Here's how the part is built. I have some questions about the finished solid (model axes, mm). Round coordinates to 2 decimals unless told otherwise and drop trailing zeros. Put each result on its own line as item: value. Start each with the question number.
1) Will this pin go through, and if not, where does the flat tip stop? P1, Ø2.5, axis at x = -86.21, z = 15.12, coming from the +Y side.
2) If I drill on line 1 along X through (y, z) = (-2.4, -26.5); line 2 along Z through (x, y) = (155, -0.95); line 3 along X through (y, z) = (-0.35, 70), over which ranges is the centre line in solid material (lowest first)? Write a range as [from, to].
3) I want a section at A-A, the plane y = -1.65. Give the number of separate pieces and of enclosed holes in the cut face, then the cut area to 3 significant figures.
from build123d import *

# Parameters (mm, degrees)
F0_R     = 1.89865
F1_DEPTH = 3.175


with BuildPart() as f1:
    # F0 (on Front) → F1 (new body)
    with BuildSketch(Plane.XZ):
        with BuildLine():
            Line((200.025, 95.25), (-200.025, 95.25))
            ThreePointArc((-200.025, 95.25), (-202.2700640303, 94.3200640303), (-203.2, 92.075))
            Line((-203.2, 92.075), (-203.2, -92.075))
            ThreePointArc((-203.2, -92.075), (-202.2700640303, -94.3200640303), (-200.025, -95.25))
            Line((-200.025, -95.25), (200.025, -95.25))
            ThreePointArc((200.025, -95.25), (202.2700640303, -94.3200640303), (203.2, -92.075))
            Line((203.2, -92.075), (203.2, 92.075))
            ThreePointArc((203.2, 92.075), (202.2700640303, 94.3200640303), (200.025, 95.25))
        make_face()
        with Locations((-152.4, -82.55)):
            Circle(F0_R, mode=Mode.SUBTRACT)
        with Locations((-101.6, -82.55)):
            Circle(F0_R, mode=Mode.SUBTRACT)
        with Locations((-150.2112307024, -64.8801388249)):
            Circle(F0_R, mode=Mode.SUBTRACT)
        with Locations((-50.8, -82.55)):
            Circle(F0_R, mode=Mode.SUBTRACT)
        with Locations((0, -82.55)):
            Circle(F0_R, mode=Mode.SUBTRACT)
        with BuildLine():
            ThreePointArc((-84.3125807024, -64.8801388249), (-86.2112307024, -66.7787888249), (-88.1098807024, -64.8801388249))
            ThreePointArc((-88.1098807024, -64.8801388249), (-86.2112307024, -62.9814888249), (-84.3125807024, -64.8801388249))
        make_face(mode=Mode.SUBTRACT)
        with BuildLine():
            ThreePointArc((-188.1665156039, -0.0463944584), (-187.2365796342, 2.1986695719), (-184.9915156039, 3.1286055416))
            Line((-184.9915156039, 3.1286055416), (-165.9415156039, 3.1286055416))
            ThreePointArc((-165.9415156039, 3.1286055416), (-163.6964515737, 2.1986695719), (-162.7665156039, -0.0463944584))
            Line((-162.7665156039, -0.0463944584), (-162.7665156039, -50.8463944584))
            ThreePointArc((-162.7665156039, -50.8463944584), (-163.6964515737, -53.0914584887), (-165.9415156039, -54.0213944584))
            Line((-165.9415156039, -54.0213944584), (-184.9915156039, -54.0213944584))
            ThreePointArc((-184.9915156039, -54.0213944584), (-187.2365796342, -53.0914584887), (-188.1665156039, -50.8463944584))
            Line((-188.1665156039, -50.8463944584), (-188.1665156039, -0.0463944584))
        make_face(mode=Mode.SUBTRACT)
        with BuildLine():
            ThreePointArc((-72.1112307024, 0.5198611751), (-71.1812947327, 2.7649252054), (-68.9362307024, 3.6948611751))
            Line((-68.9362307024, 3.6948611751), (-49.8862307024, 3.6948611751))
            ThreePointArc((-49.8862307024, 3.6948611751), (-47.6411666721, 2.7649252054), (-46.7112307024, 0.5198611751))
            Line((-46.7112307024, 0.5198611751), (-46.7112307024, -50.2801388249))
            ThreePointArc((-46.7112307024, -50.2801388249), (-47.6411666721, -52.5252028551), (-49.8862307024, -53.4551388249))
            Line((-49.8862307024, -53.4551388249), (-68.9362307024, -53.4551388249))
            ThreePointArc((-68.9362307024, -53.4551388249), (-71.1812947327, -52.5252028551), (-72.1112307024, -50.2801388249))
            Line((-72.1112307024, -50.2801388249), (-72.1112307024, 0.5198611751))
        make_face(mode=Mode.SUBTRACT)
        with Locations((50.8, -82.55)):
            Circle(F0_R, mode=Mode.SUBTRACT)
        with Locations((101.6, -82.55)):
            Circle(F0_R, mode=Mode.SUBTRACT)
        with Locations((62.75, -63.5)):
            Circle(F0_R, mode=Mode.SUBTRACT)
        with Locations((152.4, -82.55)):
            Circle(F0_R, mode=Mode.SUBTRACT)
        with Locations((158.75, -63.5)):
            Circle(F0_R, mode=Mode.SUBTRACT)
        with BuildLine():
            ThreePointArc((18.3, -12.7), (19.2299359697, -10.4549359697), (21.475, -9.525))
            Line((21.475, -9.525), (46.875, -9.525))
            ThreePointArc((46.875, -9.525), (49.1200640303, -10.4549359697), (50.05, -12.7))
            Line((50.05, -12.7), (50.05, -47.625))
            ThreePointArc((50.05, -47.625), (49.1200640303, -49.8700640303), (46.875, -50.8))
            Line((46.875, -50.8), (21.475, -50.8))
            ThreePointArc((21.475, -50.8), (19.2299359697, -49.8700640303), (18.3, -47.625))
            Line((18.3, -47.625), (18.3, -12.7))
        make_face(mode=Mode.SUBTRACT)
        with BuildLine():
            ThreePointArc((196.85, -35.375), (195.9200640303, -37.6200640303), (193.675, -38.55))
            Line((193.675, -38.55), (180.975, -38.55))
            ThreePointArc((180.975, -38.55), (178.7299359697, -37.6200640303), (177.8, -35.375))
            Line((177.8, -35.375), (177.8, -3.625))
            ThreePointArc((177.8, -3.625), (178.7299359697, -1.3799359697), (180.975, -0.45))
            Line((180.975, -0.45), (193.675, -0.45))
            ThreePointArc((193.675, -0.45), (195.9200640303, -1.3799359697), (196.85, -3.625))
            Line((196.85, -3.625), (196.85, -35.375))
        make_face(mode=Mode.SUBTRACT)
        with Locations((-150.2112307024, 15.1198611751)):
            Circle(F0_R, mode=Mode.SUBTRACT)
        with Locations((-86.2112307024, 15.1198611751)):
            Circle(F0_R, mode=Mode.SUBTRACT)
        with Locations((62.75, 24.5)):
            Circle(F0_R, mode=Mode.SUBTRACT)
        with Locations((158.75, 24.5)):
            Circle(F0_R, mode=Mode.SUBTRACT)
        with BuildLine():
            Line((155.575, 49.9), (65.925, 49.9))
            ThreePointArc((65.925, 49.9), (63.6799359697, 50.8299359697), (62.75, 53.075))
            Line((62.75, 53.075), (62.75, 72.125))
            ThreePointArc((62.75, 72.125), (63.6799359697, 74.3700640303), (65.925, 75.3))
            Line((65.925, 75.3), (155.575, 75.3))
            ThreePointArc((155.575, 75.3), (157.8200640303, 74.3700640303), (158.75, 72.125))
            Line((158.75, 72.125), (158.75, 53.075))
            ThreePointArc((158.75, 53.075), (157.8200640303, 50.8299359697), (155.575, 49.9))
        make_face(mode=Mode.SUBTRACT)
    extrude(amount=F1_DEPTH)


solid = f1.part
Findings:
1. P1: passes through
2. line 1: x = [-203.2, -188.17], [-162.77, -72.11], [-46.71, 18.3], [50.05, 177.8], [196.85, 203.2]
2. line 2: z = [-95.25, 49.9], [75.3, 95.25]
2. line 3: x = [-203.2, 62.75], [158.75, 203.2]
3. separate pieces: 1
3. enclosed holes: 20
3. area: 69,900 mm2
